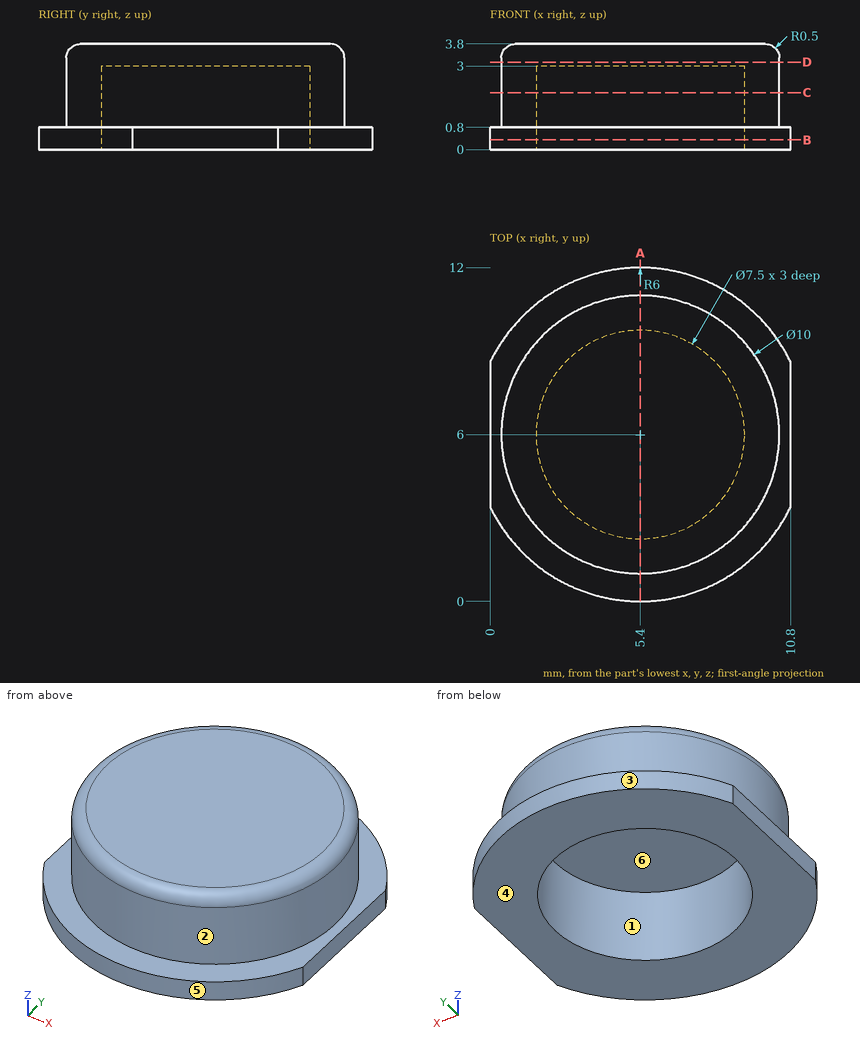
Part print with two shaded views. Sizes in mm from the minimum x, y, z corner. A direction names the side the tool comes from. Round coordinates to 2 decimals unless told otherwise and drop trailing zeros. Write each loop counter-clockwise with the first axis right and the second up, starting at its lowest first coordinate (ties: lowest second). Pieces come first, ordered by that corner, then holes. Notation, with made-up numbers: M 31.25,75.5 L 90.25,75.5 A13 ccw 90.25,94.5 Z; hole C -36,-6 d7. An arc over 180 degrees is marked long. Put each result on its own line as item: value. Start each with the question number.
1) Saw through at C-C, the plane z = 2.05. Write the cut outline in (x, y).
2) Saw through at D-D, the plane z = 3.15. Write the cut outline in (x, y), and give its area (3 significant figures).
3) Saw through at A-A, the plane x = 5.4. Write the cut outline in (y, z), and give its area (3 significant figures).
4) Drill centre lines: probe 1 along Y at (x, z) = (5.4, 1.75); probe 2 along Z at (x, y) = (10.5, 6.75); probe 3 along Z at (x, y) = (3.75, 2.75). Where is each one in solid material? Low to high. Write a range as [from, to].
5) Pin check, flat tips, straight feed: pin 1 Ø2 at (x, y) = (5.5, 7) entering from -Z; pin 2 Ø2 at (y, z) = (8, 2.5) entering from +X. Stop position of each tip, or through.
6) 3-axis set-ups, long thin cutter, end or side, ignore diameter. For the marked faces 1, 2 and 3: which of +Z, -Z, +X, -X, +Y, -Y reach the whole face in a straight line?
7) Pull direction X, two halves, no side cores. Call the marked faces 4, 5 and 6: pulls with the +X half, pulls with the -X half, needs draft (parallel to the pull), parting line crosses it, or undercut.
8) Saw through at B-B, the plane z = 0.35. Write the cut outline in (x, y), and give its area (3 significant figures).
Resolved:
1. outline: C 5.4,6 d10; hole C 5.4,6 d7.5
2. outline: C 5.4,6 d10
2. area: 78.5 mm²
3. outline: M 0,0 L 2.25,0 L 2.25,3 L 9.75,3 L 9.75,0 L 12,0 L 12,0.8 L 11,0.8 L 11,3.3 A0.5 ccw 10.5,3.8 L 1.5,3.8 A0.5 ccw 1,3.3 L 1,0.8 L 0,0.8 Z
3. area: 17.0 mm²
4. probe 1: [1, 2.25], [9.75, 11]
4. probe 2: [0, 0.8]
4. probe 3: [3, 3.8]
5. pin 1: z = 3
5. pin 2: x = 10.3
6. face 1: -Z
6. face 2: +Z
6. face 3: +Z, -Z, +Y
7. face 4: needs draft
7. face 5: parting line crosses it
7. face 6: undercut
8. outline: M 0,3.38 A6 ccw 10.8,3.38 L 10.8,8.62 A6 ccw 0,8.62 Z; hole C 5.4,6 d7.5
8. area: 64.7 mm²
